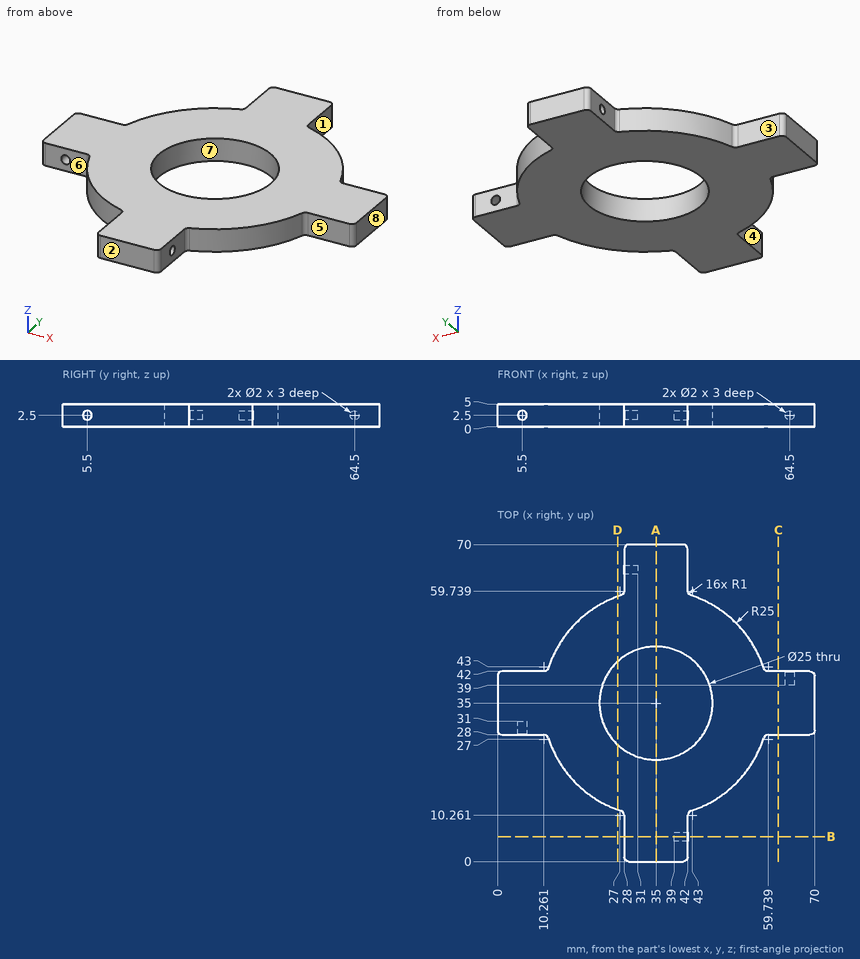
Job drawing, mm, ordinate dimensions from the low corner. One solid piece. A direction names the side the tool comes from. Round coordinates to 2 decimals unless told otherwise and drop trailing zeros. Write each loop counter-clockwise with the first axis right and the second up, starting at its lowest first coordinate (ties: lowest second). Pieces come first, ordered by that corner, then holes.
1) 3-axis set-ups, long thin cutter, end or side, ignore diameter. For the marked faces 1, 2, 3, 4 and 5: which of +Z, -Z, +X, -X, +Y, -Y reach the whole face in a straight line?
2) Drill centre lines: probe 1 along X at (y, z) = (35.5, 1.75); probe 2 along Y at (x, z) = (29.95, 2.5) (1 decimal); probe 3 along Y at (x, z) = (41.05, 2.5). Where is each one in solid material? Low to high.
3) Mould opens along X. For the marked faces 6, 7 and 8 say: +X half, -X half, draft (parallel to the pull), parting line (faces both ways), or undercut.
4) Band-saw the part on D-D, the plane x = 26.5. List the corners of the cut face in (y, z) (1 decimal).
5) Band-saw the part on A-A, the plane x = 35. List the corners of the cut face in (y, z).
6) Pin check, flat tips, straight feed: pin 1 (0.6 mm diameter, centred on x = 65, z = 2.5, fed in from +Y); pin 2 (1 mm diameter, centred on y = 14, z = 3, fed in from -X); pin 3 (1.5 mm diameter, centred on y = 7.5, z = 2, fed in from +X); pin 4 (22.5 mm diameter, centred on x = 35, y = 35, fed in from -Z). Stop position of each tip, or through.
7) Band-saw the part on B-B, the plane y = 5.5. List the corners of the cut face in (x, z).
8) Band-saw the part on C-C, the plane x = 62. List the corners of the cut face in (y, z).
Ans:
1. face 1: +Z, -Z, +X, +Y
1. face 2: +Z, -Z, +X, -X, -Y
1. face 3: +Z, -Z, -X, +Y
1. face 4: +Z, -Z, -X, -Y
1. face 5: +Z, -Z, +X, -Y
2. probe 1: x = 0 to 22.51, 47.49 to 70
2. probe 2: y = 0 to 23.6, 46.4 to 63.5, 65.5 to 70
2. probe 3: y = 0 to 4.5, 6.5 to 24.06, 45.94 to 70
3. face 6: draft
3. face 7: undercut
3. face 8: +X half
4. outline: (11.5, 0) - (25.8, 0) - (25.8, 5) - (11.5, 5) - close; (44.2, 0) - (58.5, 0) - (58.5, 5) - (44.2, 5) - close
5. outline: (0, 0) - (22.5, 0) - (22.5, 5) - (0, 5) - close; (47.5, 0) - (70, 0) - (70, 5) - (47.5, 5) - close
6. pin 1: stops at y = 39
6. pin 2: stops at x = 20.69
6. pin 3: stops at x = 42
6. pin 4: passes through
7. outline: (28, 0) - (42, 0) - (42, 1.5) - (39, 1.5) - (39, 3.5) - (42, 3.5) - (42, 5) - (28, 5) - close
8. outline: (28, 0) - (42, 0) - (42, 5) - (28, 5) - close
